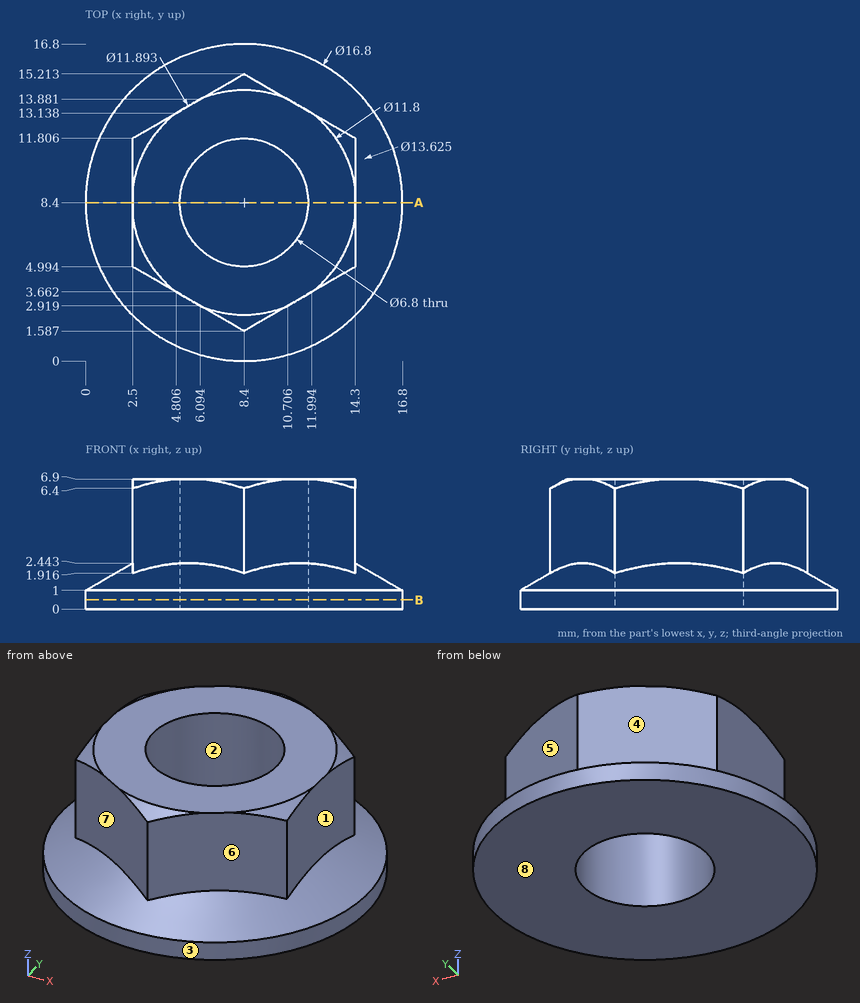
Geometry: see drawing. Coordinates: mm, zero at the bounding-box minimum. A direction names the side the tool comes from. Give positions to 0.01 mm unless a question says otherwise; leave off trailing zeros. Write each loop counter-clockwise with the first axis right and the second up, starting at its lowest first coordinate (ties: lowest second). Pieces come first, ordered by that corner, then holes. Notation, with made-up numbers: (78.5, 62) -> (95.5, 62) arc R13 cw to (95.5, 73) -> close; hole circle Ø1 at (17, 75.5). An arc over 180 degrees is marked (long way). Use one line per item in the form item = value. Start each with the question number.
1) Ray query, probe 1 along X at (y, z) = (8.5, 5.5); probe 2 along X at (y, z) = (5.75, 4.25); probe 3 along Y at (x, z) = (6, 0.75). Return the intervals inside material, ascending. Write a range as from..to.
2) Pin query (flat end, axial travel): pin 1 (2.5 mm diameter, centred on y = 8.5, z = 5, fed in from +X); pin 2 (1.5 mm diameter, centred on x = 8.5, z = 4.5, fed in from +Y). Return the tip coordinate at first contact, or that it passes through.
3) Section query B-B on z = 0.5. Return the cut outline in (x, y).
4) Set-up query: the marked faces 4, 5, 6, 7 and 8. Return all of +Z, -Z, +X, -X, +Y, -Y with unobstructed straight access to the full face (end or side cutting, diameter ignored); none if empty.
5) Draft query along Y for the marked faces 1, 2 and 3. Return one class per face: pulls with the +Y half, pulls with the -Y half, needs draft (parallel to the pull), parting line crosses it, or undercut.
6) Section query A-A on y = 8.4. Return the cut outline in (x, z).
Outcome:
q1.probe_1 = 2.5..5, 11.8..14.3
q1.probe_2 = 2.5..6.27, 10.53..14.3
q1.probe_3 = 0.35..5.99, 10.81..16.45
q2.pin_1 = 14.3
q2.pin_2 = 15.21
q3.outline = circle Ø16.8 at (8.4, 8.4); hole circle Ø6.8 at (8.4, 8.4)
q4.face_4 = +Z, -X, +Y
q4.face_5 = +Z, +X, +Y
q4.face_6 = +Z, +X, -Y
q4.face_7 = +Z, -X, -Y
q4.face_8 = -Z, +X, -X, +Y, -Y
q5.face_1 = needs draft
q5.face_2 = undercut
q5.face_3 = parting line crosses it
q6.outline = (0, 0) -> (5, 0) -> (5, 6.9) -> (2.5, 6.9) -> (2.5, 2.44) -> (0, 1) -> close; (11.8, 0) -> (16.8, 0) -> (16.8, 1) -> (14.3, 2.44) -> (14.3, 6.9) -> (11.8, 6.9) -> close
